```python
from build123d import *

# Parameters (mm, degrees)
SKETCH1_W           = 1000
SKETCH1_H           = 100
BOSS_EXTRUDE1_DEPTH = 15
SKETCH2_W           = 35
SKETCH2_H           = 67
CUT_EXTRUDE1_DEPTH  = 15
SKETCH4_W           = 35
SKETCH4_H           = 10
CUT_EXTRUDE2_DEPTH  = 100
SKETCH5_W           = 15
SKETCH5_H           = 67
CUT_EXTRUDE4_DEPTH  = 100


with BuildPart() as part:
    # Sketch1 → Boss-Extrude1 (new body)
    with BuildSketch(Plane(origin=(0, 0, 0), x_dir=(1, 0, 0), z_dir=(0, 1, 0))):
        with Locations((500, 50)):
            Rectangle(SKETCH1_W, SKETCH1_H)
    extrude(amount=BOSS_EXTRUDE1_DEPTH)

    # Sketch2 → Cut-Extrude1 (cut)
    with BuildSketch(Plane(origin=(0, 15, 0), x_dir=(1, 0, 0), z_dir=(0, 1, 0))):
        with Locations((752.5, 48.5)):
            Rectangle(SKETCH2_W, SKETCH2_H)
    extrude(amount=-CUT_EXTRUDE1_DEPTH, mode=Mode.SUBTRACT)

    # Sketch4 → Cut-Extrude2 (cut)
    with BuildSketch(Plane.XY):
        with Locations((807.5, 5)):
            Rectangle(SKETCH4_W, SKETCH4_H)
    extrude(amount=-CUT_EXTRUDE2_DEPTH, mode=Mode.SUBTRACT)

    # Sketch5 → Cut-Extrude4 (cut)
    with BuildSketch(Plane(origin=(0, 15, 0), x_dir=(1, 0, 0), z_dir=(0, 1, 0))):
        with Locations((802.5, 49.5)):
            Rectangle(SKETCH5_W, SKETCH5_H)
    extrude(amount=-CUT_EXTRUDE4_DEPTH, mode=Mode.SUBTRACT)


solid = part.part
```
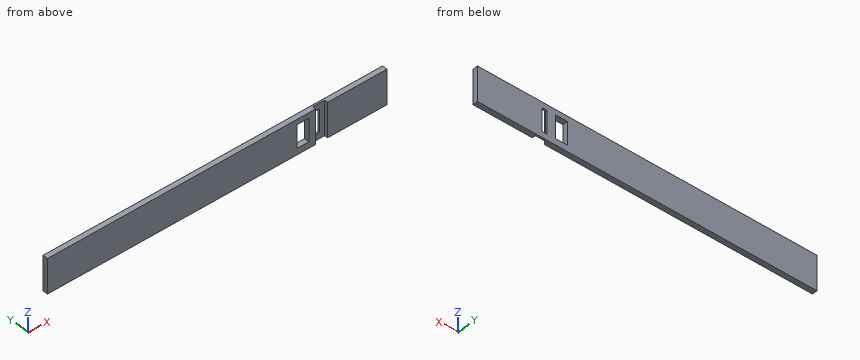
For this review, take the finished solid that the model builds, in its own axes (mm). Give positions to 0.01 mm unless a question says otherwise; leave off trailing zeros. Order: outer loops, then holes, each group sorted by start corner. A loop starts at its lowest first (then second) coordinate and runs counter-clockwise, first axis right, second up.
1) Take a section at A-A (z = -51). Give the boundary of the cut face in (x, y), then the cut area to 4 significant figures.
2) Wall thickness on line 1 (X direction, y = 8.25, z = -33); line 2 (X direction, y = 11.5, z = -25.5); line 3 (X direction, y = 7.5, z = -83): over which ranges is each line inside the solid? List them lowest first.
3) Insertion check: pin 1 (6 mm diameter, centred on x = 731.5, z = -18.5, fed in from -Y); pin 2 (17.5 mm diameter, centred on x = 807.5, z = -47, fed in from -Y). Each pin has a flat end and moves straight along its axis. Give the tip position at first contact, or say it passes through.
4) Take a section at B-B (y = 4.5). Give the boundary of the cut face in (x, z), then the cut area to 3 significant figures.
Derived:
1. outline: (0, 0) - (735, 0) - (735, 15) - (0, 15) - close; (770, 0) - (790, 0) - (790, 10) - (795, 10) - (795, 15) - (770, 15) - close; (810, 10) - (825, 10) - (825, 0) - (1000, 0) - (1000, 15) - (810, 15) - close
1. area: 14,050 mm2
2. line 1: x = 0 to 735, 770 to 790, 825 to 1000
2. line 2: x = 0 to 735, 770 to 795, 810 to 1000
2. line 3: x = 0 to 790, 825 to 1000
3. pin 1: stops at y = 0
3. pin 2: stops at y = 10
4. outline: (0, -100) - (790, -100) - (790, 0) - (0, 0) - close; (825, -100) - (1000, -100) - (1000, 0) - (825, 0) - close; hole (735, -82) - (770, -82) - (770, -15) - (735, -15) - close
4. area: 94,200 mm2
